from build123d import *

# Parameters (mm, degrees)
CROQUIS1_W              = 54
CROQUIS1_H              = 51
CROQUIS1_R              = 3.75
SALIENTE_EXTRUIR1_DEPTH = 4
CROQUIS2_W              = 32
CROQUIS2_H              = 51
SALIENTE_EXTRUIR2_DEPTH = 1


with BuildPart() as part:
    # Croquis1 → Saliente-Extruir1 (new body)
    with BuildSketch(Plane.XY):
        Rectangle(CROQUIS1_W, CROQUIS1_H)
        with Locations((-21.5, 12.5)):
            Circle(CROQUIS1_R, mode=Mode.SUBTRACT)
        with Locations((21.5, 12.5)):
            Circle(CROQUIS1_R, mode=Mode.SUBTRACT)
        with Locations((21.5, -9.5)):
            Circle(CROQUIS1_R, mode=Mode.SUBTRACT)
        with Locations((-21.5, -9.5)):
            Circle(CROQUIS1_R, mode=Mode.SUBTRACT)
    extrude(amount=-SALIENTE_EXTRUIR1_DEPTH)

    # Croquis2 → Saliente-Extruir2 (add)
    with BuildSketch(Plane.XY):
        Rectangle(CROQUIS2_W, CROQUIS2_H)
    extrude(amount=SALIENTE_EXTRUIR2_DEPTH)


solid = part.part
CAD build for the part. Positions are in the model's coordinates, mm. A direction names the side the tool comes from. Give positions to 0.01 mm unless a question says otherwise; leave off trailing zeros. Order: outer loops, then holes, each group sorted by start corner. A loop starts at its lowest first (then second) coordinate and runs counter-clockwise, first axis right, second up. Notation, with made-up numbers: (-25, 24) - (0, 24) arc R10 cw to (0, 37) - close; hole circle Ø6 at (25.25, -13.75). An arc over 180 degrees is marked (long way). Write each question's results on one line, items separated by ' | '.
1. Pull direction X, two halves, no side cores. Call faces 1 (the face through (-19.48, 15.66, -1.97)), 2 (the face through (0, -25.5, -1)), 3 (the face through (27, 0, -2)): released by +X, released by -X, zero draft, split by the parting line, or undercut.
Calculated:
face 1: undercut | face 2: zero draft | face 3: released by +X
2. Probe L1, parallel to Y at x = -21.5, z = -3.05; L2, parallel to X at y = 15, z = -3.2; L3, parallel to X at y = 10.5, z = -2.95. List the from-to ranges inside material, lowest first. Write a range as from..to.
Calculated:
L1: y = -25.5..-13.25, -5.75..8.75, 16.25..25.5 | L2: x = -27..-24.3, -18.7..18.7, 24.3..27 | L3: x = -27..-24.67, -18.33..18.33, 24.67..27
3. Saw through at B-B on y = -6.5. List the corners of the cut face in (x, z), and give its area (3 significant figures).
Calculated:
outline: (-27, -4) - (-23.75, -4) - (-23.75, 0) - (-27, 0) - close; (-19.25, -4) - (19.25, -4) - (19.25, 0) - (16, 0) - (16, 1) - (-16, 1) - (-16, 0) - (-19.25, 0) - close; (23.75, -4) - (27, -4) - (27, 0) - (23.75, 0) - close | area: 212 mm2
4. 3-axis set-ups, long thin cutter, end or side, ignore diameter. For faces 4 (the face through (-27, 0, -2)), 5 (the face through (21, 0, 0)), 6 (the face through (-22, 0, 0)): which of +Z, -Z, +X, -X, +Y, -Y reach the whole face in a straight line?
Calculated:
face 4: +Z, -Z, -X, +Y, -Y | face 5: +Z, +X, +Y, -Y | face 6: +Z, -X, +Y, -Y
5. Saw through at D-D on y = -18. List the corners of the cut face in (x, z).
Calculated:
outline: (-27, -4) - (27, -4) - (27, 0) - (16, 0) - (16, 1) - (-16, 1) - (-16, 0) - (-27, 0) - close
6. Saw through at C-C on z = -3.4. List the corners of the cut face in (x, y).
Calculated:
outline: (-27, -25.5) - (27, -25.5) - (27, 25.5) - (-27, 25.5) - close; hole circle Ø7.5 at (-21.5, -9.5); hole circle Ø7.5 at (-21.5, 12.5); hole circle Ø7.5 at (21.5, -9.5); hole circle Ø7.5 at (21.5, 12.5)
7. Pin check, flat tip, straight feed: pin 1 (5.5 mm diameter, centred on x = 24, y = 9.5, fed in from +Z). Stop position of the tip, or through.
Calculated:
pin 1: stops at z = 0
8. Saw through at A-A on x = 21.5. List the corners of the cut face in (y, z), and give its area (3 significant figures).
Calculated:
outline: (-25.5, -4) - (-13.25, -4) - (-13.25, 0) - (-25.5, 0) - close; (-5.75, -4) - (8.75, -4) - (8.75, 0) - (-5.75, 0) - close; (16.25, -4) - (25.5, -4) - (25.5, 0) - (16.25, 0) - close | area: 144 mm2
